```python
from build123d import *

# Parameters (mm, degrees)
SKETCH1_W           = 32
SKETCH1_H           = 65
BOSS_EXTRUDE1_DEPTH = 40
SKETCH2_W           = 32
SKETCH2_H           = 52.3
CUT_EXTRUDE1_DEPTH  = 37.7
BOSS_EXTRUDE4_DEPTH = 2.3
SKETCH3_7_R         = 2
SKETCH3_7_R_2       = 1.25
CUT_EXTRUDE3_DEPTH  = 2.3


with BuildPart() as part:
    # Sketch1 → Boss-Extrude1 (new body)
    with BuildSketch(Plane.XY):
        Rectangle(SKETCH1_W, SKETCH1_H)
    extrude(amount=-BOSS_EXTRUDE1_DEPTH)

    # Sketch2 → Cut-Extrude1 (cut)
    with BuildSketch(Plane(origin=(0, 0, -40), x_dir=(-1, 0, 0), z_dir=(0, 0, -1))):
        Rectangle(SKETCH2_W, SKETCH2_H)
    extrude(amount=-CUT_EXTRUDE1_DEPTH, mode=Mode.SUBTRACT)

    # Sketch3 → Boss-Extrude4 (add)
    with BuildSketch(Plane.XY):
        with BuildLine():
            Line((16, -32.5), (-16, -32.5))
            Line((-16, -32.5), (-16, -11))
            ThreePointArc((-16, -11), (-27, 0), (-16, 11))
            Line((-16, 11), (-16, 32.5))
            Line((-16, 32.5), (16, 32.5))
            Line((16, 32.5), (16, 11))
            ThreePointArc((16, 11), (27, 0), (16, -11))
            Line((16, -11), (16, -32.5))
        make_face()
    extrude(amount=-BOSS_EXTRUDE4_DEPTH)

    # Sketch3_7 → Cut-Extrude3 (cut)
    with BuildSketch(Plane.XY):
        with BuildLine():
            ThreePointArc((-22.75, 0), (-20, -2.75), (-17.25, 0))
            ThreePointArc((-17.25, 0), (-20, 2.75), (-22.75, 0))
        make_face()
        with BuildLine():
            ThreePointArc((17.25, 0), (20, -2.75), (22.75, 0))
            ThreePointArc((22.75, 0), (20, 2.75), (17.25, 0))
        make_face()
        with Locations((-12.5, 12.5)):
            Circle(SKETCH3_7_R)
        with BuildLine():
            ThreePointArc((-1.734657981, -7.142370873), (-0.873519914, -7.297908122), (0, -7.35))
            Line((0, -7.35), (0, 7.35))
            ThreePointArc((0, 7.35), (-5.778072177, 4.542728467), (-7.142370873, -1.734657981))
            ThreePointArc((-7.142370873, -1.734657981), (-7.092420905, -1.861539458), (-7.010048694, -1.970207427))
            Line((-7.010048694, -1.970207427), (-1.970207427, -7.010048694))
            ThreePointArc((-1.970207427, -7.010048694), (-1.861539458, -7.092420905), (-1.734657981, -7.142370873))
        make_face()
        with Locations((9.000000134, 0)):
            Circle(SKETCH3_7_R_2)
        with BuildLine():
            ThreePointArc((0, -7.750000134), (-1.25, -9.000000134), (0, -10.250000134))
            Line((0, -10.250000134), (0, -7.750000134))
        make_face()
        with BuildLine():
            Line((0, -7.750000134), (0, -10.250000134))
            ThreePointArc((0, -10.250000134), (0.883883476, -9.883883611), (1.25, -9.000000134))
            ThreePointArc((1.25, -9.000000134), (0.883883476, -8.116116658), (0, -7.750000134))
        make_face()
        with Locations((-9.000000134, 0)):
            Circle(SKETCH3_7_R_2)
        with BuildLine():
            ThreePointArc((1.25, 9.000000134), (0.883883476, 9.883883611), (0, 10.250000134))
            Line((0, 10.250000134), (0, 7.750000134))
            ThreePointArc((0, 7.750000134), (0.883883476, 8.116116658), (1.25, 9.000000134))
        make_face()
        with BuildLine():
            Line((0, 7.750000134), (0, 10.250000134))
            ThreePointArc((0, 10.250000134), (-1.25, 9.000000134), (0, 7.750000134))
        make_face()
        with Locations((12.5, 12.5)):
            Circle(SKETCH3_7_R)
        with Locations((-12.5, -12.5)):
            Circle(SKETCH3_7_R)
        with Locations((12.5, -12.5)):
            Circle(SKETCH3_7_R)
        with BuildLine():
            Line((0, 7.35), (0, -7.35))
            ThreePointArc((0, -7.35), (5.778072177, -4.542728467), (7.142370873, 1.734657981))
            ThreePointArc((7.142370873, 1.734657981), (7.092420905, 1.861539458), (7.010048694, 1.970207427))
            Line((7.010048694, 1.970207427), (1.970207427, 7.010048694))
            Line((1.970207427, 7.010048694), (1.734657981, 7.142370873))
            ThreePointArc((1.734657981, 7.142370873), (0.873519914, 7.297908122), (0, 7.35))
        make_face()
    extrude(amount=-CUT_EXTRUDE3_DEPTH, mode=Mode.SUBTRACT)


solid = part.part
```
Can you work these out from the model? Positions are in its coordinate system, mm. A direction names the side the tool comes from. Round coordinates to 2 decimals unless told otherwise and drop trailing zeros. Loops run counter-clockwise (first coordinate to the right, second up) from the corner with the lowest first, then second, coordinate; pieces in that order, holes last.
Item 1: Will these pins go through, and if not, where does the flat tip stop? pin 1 Ø23.5 at (y, z) = (22.5, -29.5) entering from -X; pin 2 Ø4.5 at (x, y) = (-20, 0) entering from +Z; pin 3 Ø1.5 at (x, y) = (-0.5, -20.5) entering from -Z; pin 4 Ø17 at (y, z) = (20, -29) entering from +X.
Item 2: Please list where these lines run through material, in increasing order: L1, parallel to Y at x = -7, z = -8; L2, parallel to Y at x = -20, z = -1.8; L3, parallel to Z at x = -9.5, y = -7.
Item 3: If we mould it in two halves opening along X, with no side actions, what happens to faces 5 (the cylindrical face through (-12.76, 14.483, -1.134)), 6 (the cylindrical face through (27, 0, -1)), 7 (the cylindrical face through (12.24, 14.483, -1.134)), 8 (the flat face through (-6, 6, -2.3))? For each: +X half, -X half, draft (parallel to the pull), parting line (faces both ways), or undercut.
Item 4: Suppose I cut it at D-D, the plane y = 5. Write out the boundary of the cut face in (x, z), then the cut area to 3 significant figures.
Item 5: Which directions (+Z, -Z, +X, -X, +Y, -Y) give clear straight access to the entire face, cutting with the end or side of a thin tool? Please do faces 1 (the flat face through (16, 26.4, -15.3)), 2 (the flat face through (4.53, 4.45, -1.13)), 3 (the flat face through (0, 26.15, -21)), 4 (the flat face through (-16, -27, -15)).
Item 6: Suppose I cut it at A-A, the plane z = -24.5. Write out the boundary of the cut face in (x, y), then the cut area to 3 significant figures.
Item 7: Suppose I cut it at C-C, the plane y = 12.5. Write out the boundary of the cut face in (x, z), then the cut area to 3 significant figures.
Item 8: Suppose I cut it at B-B, the plane x = 12.5. Write out the boundary of the cut face in (y, z), then the cut area to 3 significant figures.
Reported:
1. pin 1: stops at x = -16
1. pin 2: passes through
1. pin 3: stops at z = -2.3
1. pin 4: stops at x = 16
2. L1: y = -32.5 to -26.15, 26.15 to 32.5
2. L2: y = -10.25 to -2.75, 2.75 to 10.25
2. L3: z = -2.3 to 0
3. face 5: undercut
3. face 6: +X half
3. face 7: undercut
3. face 8: draft
4. outline: (-25.8, -2.3) - (-5.39, -2.3) - (-5.39, 0) - (-25.8, 0) - close; (3.98, -2.3) - (25.8, -2.3) - (25.8, 0) - (3.98, 0) - close
4. area: 97.1 mm2
5. face 1: +Z, -Z, +X, +Y
5. face 2: +Z, -Z
5. face 3: -Z, +X, -X
5. face 4: +Z, -Z, -X, -Y
6. outline: (-16, -32.5) - (16, -32.5) - (16, -26.15) - (-16, -26.15) - close; (-16, 26.15) - (16, 26.15) - (16, 32.5) - (-16, 32.5) - close
6. area: 406 mm2
7. outline: (-16, -2.3) - (-14.5, -2.3) - (-14.5, 0) - (-16, 0) - close; (-10.5, -2.3) - (10.5, -2.3) - (10.5, 0) - (-10.5, 0) - close; (14.5, -2.3) - (16, -2.3) - (16, 0) - (14.5, 0) - close
7. area: 55.2 mm2
8. outline: (-32.5, -40) - (-26.15, -40) - (-26.15, -2.3) - (-14.5, -2.3) - (-14.5, 0) - (-32.5, 0) - close; (-10.5, -2.3) - (10.5, -2.3) - (10.5, 0) - (-10.5, 0) - close; (14.5, -2.3) - (26.15, -2.3) - (26.15, -40) - (32.5, -40) - (32.5, 0) - (14.5, 0) - close
8. area: 610 mm2
